Can you work these out from the model? Positions are in its coordinate system, mm. A direction names the side the tool comes from. Round coordinates to 2 decimals unless told otherwise and drop trailing zeros. Order: outer loops, then holes, each group sorted by start corner. A loop starts at its lowest first (then second) coordinate and runs counter-clockwise, first axis right, second up. Notation, with made-up numbers: (78.5, 66) -> (94.5, 66) arc R27 cw to (94.5, 90) -> close; hole circle Ø2 at (22.25, 84). An arc over 180 degrees is marked (long way). Use a Markdown table: item, result. Add a question column.
Q1. I need wall thicknesses on line 1 along Y through (x, z) = (41.5, 2.5); line 2 along X through (y, z) = (-1.5, -2.25); line 3 along X through (y, z) = (2.5, -2.5). Which ranges of each line are inside material? Lowest first, please. Write a range as [from, to].
Q2. For faces 1 (the face through (50, -1, -1)), 2 (the face through (25, 2, -1)), 3 (the face through (25, 0, 1)), which set-ups out of +Z, -Z, +X, -X, +Y, -Y let a thin tool reach every point of the face, with its end or its side?
Q3. If we section it at A-A on z = -4: List the corners of the cut face in (x, y) for me, plus the area to 3 significant figures.
Q4. If we section it at B-B on y = 1.5: List the corners of the cut face in (x, z) for me.
Q5. I'm going to push flat-ended pins straight in: pin 1 Ø2 at (x, z) = (51.5, 0.5) entering from +Y; pin 2 Ø3.5 at (x, z) = (12.5, -3) entering from +Y; pin 3 Ø2 at (y, z) = (-0.5, 0) entering from +X. Where does each tip first touch, or does it pass through?
```python
from build123d import *

# Parameters (mm, degrees)
BOSS_EXTRUDE1_DEPTH = 5
SKETCH2_W           = 56
SKETCH2_H           = 8
BOSS_EXTRUDE2_DEPTH = 4
SKETCH3_3_W         = 3
SKETCH3_3_H         = 8
CUT_EXTRUDE2_DEPTH  = 2
SKETCH3_W           = 3
SKETCH3_H           = 8
BOSS_EXTRUDE4_DEPTH = 5
FILLET1_R           = 0.5


with BuildPart() as part:
    # Sketch1 → Boss-Extrude1 (new body)
    with BuildSketch(Plane(origin=(0, 0, 0), x_dir=(1, 0, 0), z_dir=(0, 1, 0))):
        Polygon((0, 0), (50, 0), (0, 2), align=None)
    extrude(amount=BOSS_EXTRUDE1_DEPTH)

    # Sketch2 → Boss-Extrude2 (add)
    with BuildSketch(Plane.XZ):
        with Locations((25, -1)):
            Rectangle(SKETCH2_W, SKETCH2_H)
    extrude(amount=BOSS_EXTRUDE2_DEPTH)

    # Sketch3<3> → Cut-Extrude2 (cut)
    with BuildSketch(Plane(origin=(0, 0, 0), x_dir=(1, 0, 0), z_dir=(0, 1, 0))):
        with Locations((51.5, 1)):
            Rectangle(SKETCH3_3_W, SKETCH3_3_H)
    extrude(amount=-CUT_EXTRUDE2_DEPTH, mode=Mode.SUBTRACT)

    # Sketch3 → Boss-Extrude4 (add)
    with BuildSketch(Plane(origin=(0, 0, 0), x_dir=(1, 0, 0), z_dir=(0, 1, 0))):
        with Locations((-1.5, 1)):
            Rectangle(SKETCH3_W, SKETCH3_H)
        with Locations((51.5, 1)):
            Rectangle(SKETCH3_W, SKETCH3_H)
    extrude(amount=BOSS_EXTRUDE4_DEPTH)


with BuildPart() as boss_extrude4_kept_piece:
    # of the separate pieces the step leaves, the one the design keeps (boss_extrude4_pieces_kept)
    add(part.part.solids().sort_by_distance((0, 0, 3))[0])

    # Fillet1
    fillet1_edges = [boss_extrude4_kept_piece.edges().sort_by_distance(p)[0] for p in [
        (-3, 0.5, 3),
        (25, 5, -1),
        (-3, 0.5, -5),
        (53, -3, -5),
        (53, -3, 3),
        (-3, -4, -1),
        (25, -4, -5),
        (53, -4, -1),
        (25, -4, 3),
        (25, 0, 3),
        (51.5, -2, -5),
        (50, -1, -5),
        (53, -2, -1),
        (51.5, -2, 3),
        (50, -1, 3),
        (25, 0, -5),
        (0, 5, 1.5),
        (0, 2.5, 3),
        (0, 5, -3.5),
        (0, 2.5, -5),
        (-1.5, 5, -5),
        (-3, 5, -1),
        (-1.5, 5, 3),
        (25, 5, 0),
    ]]
    fillet(fillet1_edges, radius=FILLET1_R)


solid = boss_extrude4_kept_piece.part
```
Answer below:
| question | item | result |
|---|---|---|
| 1 | line 1 | [-4, 0] |
| 1 | line 2 | [-3, 50] |
| 1 | line 3 | [-3, 0] |
| 2 | face 1 | +Z, -Z, +X, +Y |
| 2 | face 2 | -Z, +X, +Y |
| 2 | face 3 | +Z, +X, +Y |
| 3 | outline | (-3, -3.5) arc R0.5 ccw to (-2.5, -4) -> (52.5, -4) arc R0.5 ccw to (53, -3.5) -> (53, -2.5) arc R0.5 ccw to (52.5, -2) -> (50, -2) -> (50, 0) -> (0, 0) -> (0, 4.5) arc R0.5 ccw to (-0.5, 5) -> (-2.5, 5) arc R0.5 ccw to (-3, 4.5) -> close |
| 3 | area | 233 mm² |
| 4 | outline | (-3, -4.5) arc R0.5 ccw to (-2.5, -5) -> (-0.5, -5) arc R0.5 ccw to (0, -4.5) -> (0, -2) -> (50, 0) -> (0, 0) -> (0, 2.5) arc R0.5 ccw to (-0.5, 3) -> (-2.5, 3) arc R0.5 ccw to (-3, 2.5) -> close |
| 5 | pin 1 | y = -2 |
| 5 | pin 2 | y = 4.93 |
| 5 | pin 3 | x = 50 |
